Verification items for the finished model (mm, model axes). Face numbers are marked on the shaded views. Coordinates: 2 decimals unless noted, no trailing zeros. Write each loop counter-clockwise with the first axis right and the second up, starting at its lowest first coordinate (ties: lowest second). Pieces come first, ordered by that corner, then holes. Notation, with made-up numbers: (24, 48.5) -> (52, 48.5) arc R10 ccw to (52, 53.5) -> close; hole circle Ø2 at (80, 69). An arc over 180 degrees is marked (long way). Use CSV: the item, a comma, the result in double quotes.
```python
from build123d import *

# Parameters (mm, degrees)
SKETCH1_R           = 15
BOSS_EXTRUDE1_DEPTH = 55


with BuildPart() as part:
    # Sketch1 → Boss-Extrude1 (new body)
    with BuildSketch(Plane.XY):
        with Locations((0.142780768, -8.511321707)):
            Circle(SKETCH1_R)
        with BuildLine():
            Line((2, 3.016416073), (-2, 3.016416073))
            Line((-2, 3.016416073), (-2, 0.229873324))
            ThreePointArc((-2, 0.229873324), (0.289224182, -17.510130202), (2, 0.294967904))
            Line((2, 0.294967904), (2, 3.016416073))
        make_face(mode=Mode.SUBTRACT)
    extrude(amount=BOSS_EXTRUDE1_DEPTH)


solid = part.part
```
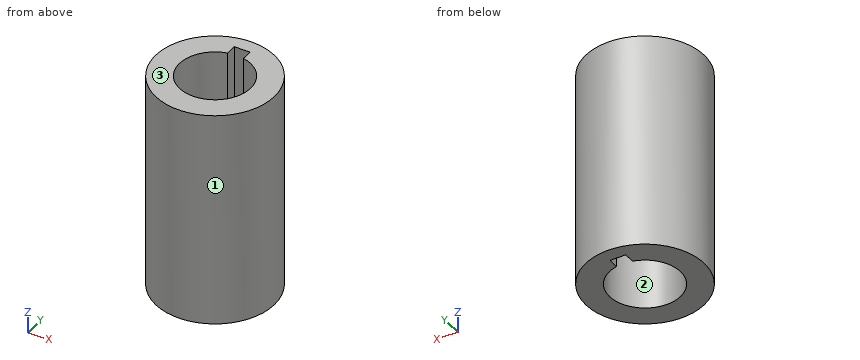
1) Cross-section at C-C (z = 41.5). Record the boundary of the cut face in (x, y).
Return value:
outline,"circle Ø30 at (0.14, -8.51); hole (-2, 0.23) arc R9 ccw (long way) to (2, 0.29) -> (2, 3.02) -> (-2, 3.02) -> close"
2) Mould release check, pull along X, two halves, no side actions. Record for the marked faces 1, 2 and 3: released by +X, released by -X, zero draft, split by the parting line, or undercut.
Return value:
face 1,"split by the parting line"
face 2,"undercut"
face 3,"zero draft"
3) Gauge pin test, flat ends, axial feed: pin 1 (3 mm diameter, centred on x = 2, z = 22, fed in from -Y); pin 2 (3 mm diameter, centred on x = 4, z = 48.5, fed in from +Y); pin 3 (1 mm diameter, centred on x = -6, z = 48, fed in from +Y). Record the tip position at first contact, or that the pin passes through.
Return value:
pin 1,"y = -23.51"
pin 2,"y = 6.3"
pin 3,"y = 5.39"
4) Cross-section at A-A (x = 6.5). Record the boundary of the cut face in (y, z).
Return value:
outline,"(-22.1, 0) -> (-14.88, 0) -> (-14.88, 55) -> (-22.1, 55) -> close; (-2.14, 0) -> (5.07, 0) -> (5.07, 55) -> (-2.14, 55) -> close"
5) Scan lines: L1, parallel to X at y = -8.75, z = 11; L2, parallel to Y at x = 0.5, z = 24; L3, parallel to X at y = -13.5, z = 52. Record each from-to range of solid material in increasing order.
Return value:
L1,"-14.86 to -8.85, 9.14 to 15.14"
L2,"-23.51 to -17.5, 3.02 to 6.48"
L3,"-14 to -7.35, 7.63 to 14.29"
6) Cross-section at B-B (y = -5.25). Record the boundary of the cut face in (x, z).
Return value:
outline,"(-14.5, 0) -> (-8.25, 0) -> (-8.25, 55) -> (-14.5, 55) -> close; (8.53, 0) -> (14.78, 0) -> (14.78, 55) -> (8.53, 55) -> close"
7) Cross-section at D-D (x = 11). Record the boundary of the cut face in (y, z).
Return value:
outline,"(-18.86, 0) -> (1.84, 0) -> (1.84, 55) -> (-18.86, 55) -> close"
